The drawing under review shows one solid part. Ordinate dimensions are in mm from its lowest x, y, z. A direction names the side the tool comes from. Coordinates: 2 decimals unless noted, no trailing zeros. Order: outer loops, then holes, each group sorted by start corner. A loop starts at its lowest first (then second) coordinate and runs counter-clockwise, first axis right, second up. Notation, with made-up numbers: (82.25, 88) - (98.25, 88) arc R15 ccw to (98.25, 103) - close; hole circle Ø7 at (0, -38.75). An arc over 180 degrees is marked (long way). Write item = value, one per line. Start each with the question number.
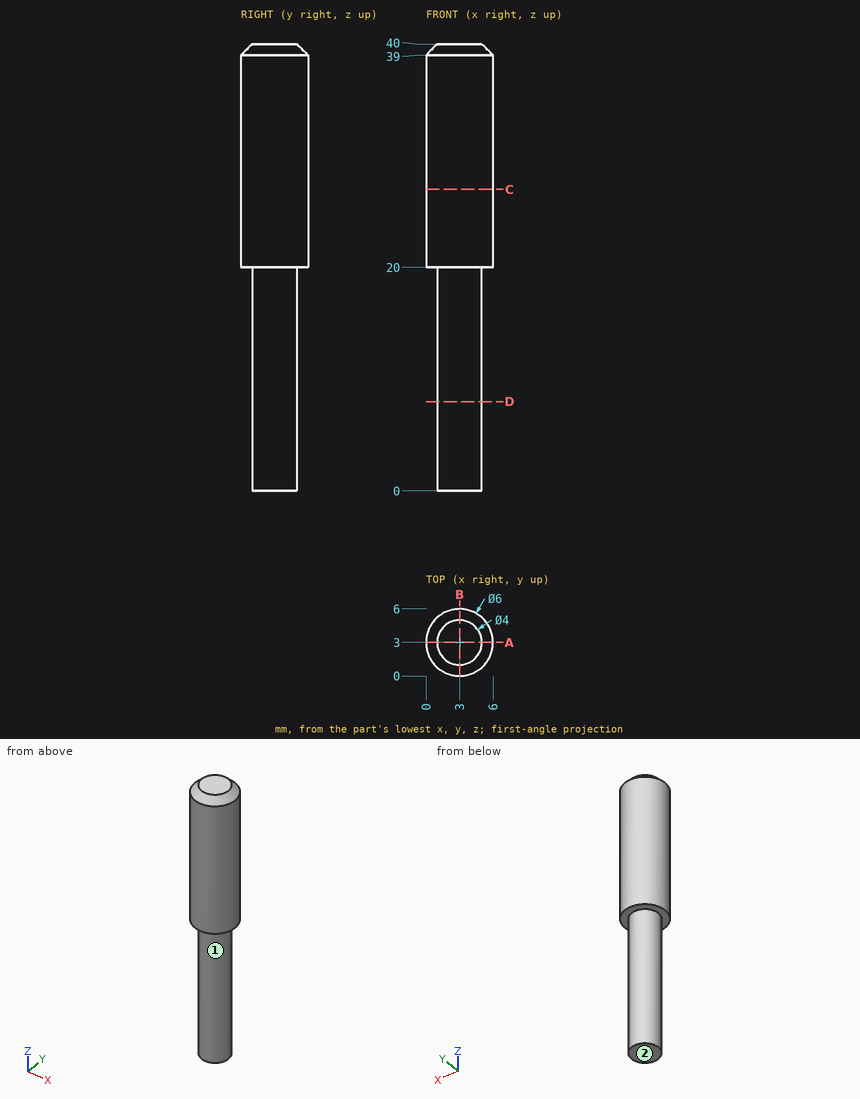
Item 1: Add section A-A on y = 3. Give the boundary of the cut face in (x, z), plus the area to 3 significant figures.
Item 2: For line 1 (Y direction, x = 3, z = 14.5); line 2 (Z direction, x = 1.4, y = 0.7); line 3 (X direction, y = 3.7, z = 29), list the stretches that pass through material, from the lowest coordinate up.
Item 3: For the marked faces 1 and 2, list the 3-axis set-ups (+Z, -Z, +X, -X, +Y, -Y) from which the entire face can be reached by the end or side of a thin tool; tool diameter is ignored.
Item 4: Add section C-C on z = 27. Give the boundary of the cut face in (x, y).
Item 5: Add section D-D on z = 8. Give the boundary of the cut face in (x, y).
Worked out:
q1.outline = (0, 20) - (1, 20) - (1, 0) - (5, 0) - (5, 20) - (6, 20) - (6, 39) - (5, 40) - (1, 40) - (0, 39) - close
q1.area = 199 mm2
q2.line_1 = 1 to 5
q2.line_2 = 20 to 39.2
q2.line_3 = 0.08 to 5.92
q3.face_1 = -Z
q3.face_2 = -Z, +X, -X, +Y, -Y
q4.outline = circle Ø6 at (3, 3)
q5.outline = circle Ø4 at (3, 3)
